Check sheet for the modelled part. Datum: model origin and axes. Units: mm. A direction names the side the tool comes from. Give positions to 0.01 mm unless a question says otherwise; leave off trailing zeros. Loops run counter-clockwise (first coordinate to the right, second up) from the corner with the lowest first, then second, coordinate; pieces in that order, holes last. Notation, with made-up numbers: M 27.5,-4 L 35.5,-4 A29 ccw 35.5,23 Z; hole C 76.5,57.25 d7. An arc over 180 degrees is marked long. Use one line per item in the form item = value.
Autodesk Inventor part; units mm, degrees
ref_plane "YZ Plane" through (0, 0, 0) normal (1, 0, 0) x (0, 1, 0)
ref_plane "XZ Plane" through (0, 0, 0) normal (0, 1, 0) x (-1, 0, 0)
ref_plane "XY Plane" through (0, 0, 0) normal (0, 0, 1) x (1, 0, 0)
sketch "Sketch1" plane through (0, 0, 0) normal (0, 1, 0) x (-1, 0, 0)
  circle A0 centre (0, 0) radius 85
  circle A1 centre (0, 0) radius 80
  dimension "d0" = 170
  dimension "d1" = 160
extrude "Extrusion1" add sketch "Sketch1" along normal blind 10 contours A0 | A1
extrude "Extrusion2" add sketch "Sketch1" along normal blind 50
sketch "Sketch2" plane through (0, 50, 0) normal (0, 1, 0) x (1, 0, 0)
  circle A0 centre (0, 0) radius 85
extrude "Extrusion3" add sketch "Sketch2" against normal blind 10
sketch "Sketch3" plane through (0, 50, 0) normal (0, 1, 0) x (1, 0, 0)
  circle A0 centre (0, 0) radius 76
  circle A1 centre (0, -76) radius 2.25
  circle A2 centre (0, 76) radius 2.25
  dimension "d8" = 152
  dimension "d9" = 4.5
  dimension "d10" = 4.5
extrude "Extrusion4" cut sketch "Sketch3" against normal blind 10 contours A2 A0 | A0 A2 | A1 A0 | A0 A1
sketch "Sketch4" plane through (0, 0, 0) normal (0, -1, 0) x (1, 0, 0)
  circle A0 centre (0, -76) radius 2.25
  circle A1 centre (0, 0) radius 76
  circle A2 centre (0, 76) radius 2.25
extrude "Extrusion5" cut sketch "Sketch4" against normal blind 10 contours A2 A1 | A1 A2
properties part number "Capsule"
1) Depth check by flat-ended pin: pin 1 Ø10 at (x, y) = (-20.5, 43) entering from -Z; pin 2 Ø3 at (x, y) = (-50, 44.5) entering from +Z; pin 3 Ø2 at (y, z) = (12, 50) entering from +X (3 decimals). Enter the tip coordinate at first touch or a pass-through.
Evaluation:
pin_1 = -83.57
pin_2 = 69.81
pin_3 = 69.455
2) Section check A-A (x = 0). Record the cut outline in (y, z).
Evaluation:
outline = M 0,-85 L 50,-85 L 50,-78.25 L 40,-78.25 L 40,-80 L 10,-80 L 10,73.75 L 0,73.75 Z; M 0,78.25 L 10,78.25 L 10,80 L 40,80 L 40,78.25 L 50,78.25 L 50,85 L 0,85 Z; M 40,-73.75 L 50,-73.75 L 50,73.75 L 40,73.75 Z
3) Release check for a two-part mould opening along Y. For faces 3 (the face through (1, 0, 1)), 4 (the face through (-0.488, 45.07, -73.804)), 5 (the face through (1, 50, 1)), 6 (the face through (1, 10, 1)) record: pulls with the +Y half, pulls with the -Y half, needs draft (parallel to the pull), parting line crosses it, or undercut.
Evaluation:
face_3 = pulls with the -Y half
face_4 = needs draft
face_5 = pulls with the +Y half
face_6 = undercut
4) Scan lines: line 1 (Z direction, x = 0, y = 44); line 2 (X direction, y = 16, z = 0); line 3 (Y direction, x = 62, z = 9). Record each from-to range of solid material in increasing order.
Evaluation:
line_1 = -85 to -78.25, -73.75 to 73.75, 78.25 to 85
line_2 = -85 to -80, 80 to 85
line_3 = 0 to 10, 40 to 50
5) Set-up check for faces 1 (the face through (-1, 40, -1)), 2 (the face through (67.453, 24.65, 51.721)): record each of +Z, -Z, +X, -X, +Y, -Y from which the full face is reachable in a straight line by a thin tool's end or side.
Evaluation:
face_1 = none
face_2 = +Y, -Y
6) Section check C-C (z = 76). Record the cut outline in (x, y), then the cut area to 3 significant figures.
Evaluation:
outline = M -38.07,0 L -2.25,0 L -2.25,10 L -24.98,10 L -24.98,40 L -2.25,40 L -2.25,50 L -38.07,50 Z; M 2.25,0 L 38.07,0 L 38.07,50 L 2.25,50 L 2.25,40 L 24.98,40 L 24.98,10 L 2.25,10 Z
area = 2,220 mm^2
7) Section check B-B (z = 0). Record the cut outline in (x, y).
Evaluation:
outline = M -85,0 L 85,0 L 85,50 L -85,50 Z; hole M -80,10 L 80,10 L 80,40 L -80,40 Z
8) Section check D-D (x = 67). Record the cut outline in (y, z), then the cut area to 3 significant figures.
Evaluation:
outline = M 0,-52.31 L 50,-52.31 L 50,52.31 L 0,52.31 Z; hole M 10,-43.71 L 40,-43.71 L 40,43.71 L 10,43.71 Z
area = 2,610 mm^2
